from build123d import *

# Parameters (mm, degrees)
SKETCH_1_W          = 40
SKETCH_1_H          = 30
SKETCH_1_W_2        = 38
SKETCH_1_H_2        = 28
EXTRUDE_1_DEPTH     = 100
SKETCH_2_R          = 1.5
CUT_EXTRUDE_1_DEPTH = 112.803398875
SKETCH_3_R          = 1.5
CUT_EXTRUDE_2_DEPTH = 112.803398875


with BuildPart() as part:
    # 草图1 → 拉伸-薄壁1 (new body)
    with BuildSketch(Plane(origin=(0, 0, 0), x_dir=(1, 0, 0), z_dir=(0, 1, 0))):
        with Locations((20, 15)):
            Rectangle(SKETCH_1_W, SKETCH_1_H)
        with Locations((20, 15)):
            Rectangle(SKETCH_1_W_2, SKETCH_1_H_2, mode=Mode.SUBTRACT)
    extrude(amount=EXTRUDE_1_DEPTH)

    # 草图2 → 切除-拉伸1 (cut, through all)
    with BuildSketch(Plane.XY):
        with Locations((5, 95)):
            Circle(SKETCH_2_R)
        with Locations((35, 95)):
            Circle(SKETCH_2_R)
        with Locations((35, 25)):
            Circle(SKETCH_2_R)
        with Locations((5, 25)):
            Circle(SKETCH_2_R)
        with Locations((5, 5)):
            Circle(SKETCH_2_R)
        with Locations((35, 5)):
            Circle(SKETCH_2_R)
    extrude(amount=-CUT_EXTRUDE_1_DEPTH, mode=Mode.SUBTRACT)

    # 草图3 → 切除-拉伸2 (cut, through all)
    with BuildSketch(Plane.ZY):
        with Locations((-25, 90)):
            Circle(SKETCH_3_R)
        with Locations((-5, 90)):
            Circle(SKETCH_3_R)
        with Locations((-25, 10)):
            Circle(SKETCH_3_R)
        with Locations((-5, 10)):
            Circle(SKETCH_3_R)
    extrude(amount=-CUT_EXTRUDE_2_DEPTH, mode=Mode.SUBTRACT)


solid = part.part
Geometry: final body of the model. Coordinates: model frame, mm. A direction names the side the tool comes from. Coordinates: 2 decimals unless noted, no trailing zeros. Order: outer loops, then holes, each group sorted by start corner. A loop starts at its lowest first (then second) coordinate and runs counter-clockwise, first axis right, second up.
(1) Draft query along Z for faces 1 (the face through (0.493, 91.487, -25.195)), 2 (the face through (33.89, 26.01, -0.49)). Return one class per face: pulls with the +Z half, pulls with the -Z half, needs draft (parallel to the pull), parting line crosses it, or undercut.
(2) Access query for faces 3 (the face through (0.49, 10.07, -26.5)), 4 (the face through (39, 49, -15)). Directions: +Z, -Z, +X, -X, +Y, -Y. A direction counts if a zero-diameter tool reaches every point of the face in a straight line with its end or side. Return the directions, or none.
(3) Section query C-C (y = 25). Return the cut outline in (x, z), plus the area to 3 significant figures.
(4) Section query A-A (z = -8.75). Return the cut outline in (x, y), plus the area to 3 significant figures.
(5) Section query D-D (x = 5). State how many separate pieces and enclosed holes the cut face has, plus the area to 3 significant figures.
(6) Section query B-B (x = 12). Return the cut outline in (y, z), plus the area to 3 significant figures.
(7) Material intervals for probe 1 along Y at (x, z) = (0.5, -25); probe 2 along Y at (x, z) = (35, -29.4); probe 3 along Z at (x, y) = (16, 61), sorted ascending.
Solution:
1. face 1: undercut
1. face 2: needs draft
2. face 3: +X, -X
2. face 4: +Y, -Y
3. outline: (0, -30) - (3.5, -30) - (3.5, -29) - (1, -29) - (1, -1) - (3.5, -1) - (3.5, 0) - (0, 0) - close; (6.5, -30) - (33.5, -30) - (33.5, -29) - (6.5, -29) - close; (6.5, -1) - (33.5, -1) - (33.5, 0) - (6.5, 0) - close; (36.5, -30) - (40, -30) - (40, 0) - (36.5, 0) - (36.5, -1) - (39, -1) - (39, -29) - (36.5, -29) - close
3. area: 124 mm2
4. outline: (0, 0) - (1, 0) - (1, 100) - (0, 100) - close; (39, 0) - (40, 0) - (40, 100) - (39, 100) - close
4. area: 200 mm2
5. separate pieces: 8
5. enclosed holes: 0
5. area: 182 mm2
6. outline: (0, -30) - (100, -30) - (100, -29) - (0, -29) - close; (0, -1) - (100, -1) - (100, 0) - (0, 0) - close
6. area: 200 mm2
7. probe 1: y = 0 to 8.5, 11.5 to 88.5, 91.5 to 100
7. probe 2: y = 0 to 3.5, 6.5 to 23.5, 26.5 to 93.5, 96.5 to 100
7. probe 3: z = -30 to -29, -1 to 0
